Build history of the part. All positions in model axes, mm. Face numbers are marked on the shaded views. A direction names the side the tool comes from. Round coordinates to 2 decimals unless told otherwise and drop trailing zeros. Order: outer loops, then holes, each group sorted by start corner. A loop starts at its lowest first (then second) coordinate and runs counter-clockwise, first axis right, second up. Notation, with made-up numbers: (46, -38) -> (62, -38) arc R19 cw to (62, -10) -> close; hole circle Ø2 at (77.5, 21). An arc over 180 degrees is marked (long way). Answer as CSV lines item,"result". Start each with the question number.
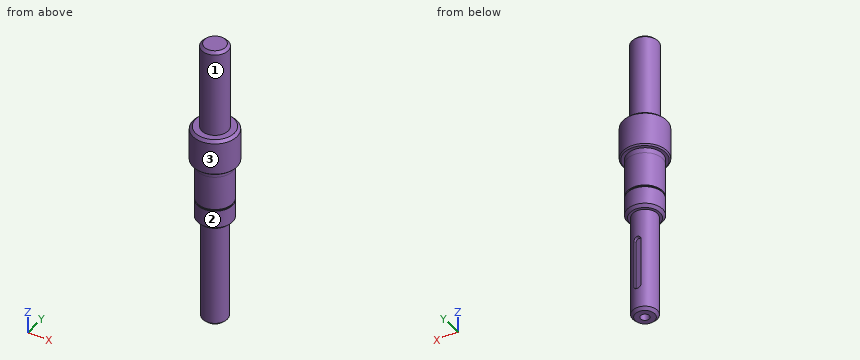
```python
from build123d import *

# Parameters (mm, degrees)
CHAMFER_1_SIZE         = 3
HOLE_WIZARD_M121_D     = 10.2
HOLE_WIZARD_M121_DEPTH = 30
HOLE_WIZARD_M121_TIP   = 3.064389157
SKETCH_4_R             = 20
SKETCH_4_R_2           = 18.75
CUT_EXTRUDE_1_DEPTH    = 2
FILLET_1_R             = 0.3
CHAMFER_2_SIZE         = 1.5
CUT_EXTRUDE_2_DEPTH    = 334.782863551
SKETCH_9_R             = 25
SKETCH_9_R_2           = 20
CUT_EXTRUDE_4_DEPTH    = 6
CHAMFER_3_SIZE         = 1.5
CHAMFER_4_SIZE         = 3


with BuildPart() as part:
    # Sketch 1 → Revolve 1 (revolve)
    with BuildSketch(Plane(origin=(0, 0, 0), x_dir=(0, 0, -1), z_dir=(1, 0, 0)), mode=Mode.PRIVATE) as revolve_1_sk:
        Polygon((0, 0), (0, 15), (100, 15), (100, 25), (147, 25), (147, 20), (211, 20), (211, 14), (331, 14), (331, 0), align=None)
    revolve(revolve_1_sk.sketch.rotate(Axis((0, 0, 0), (0, 0, -1)), 90), axis=Axis((0, 0, 0), (0, 0, -1)))

    # Chamfer 1
    chamfer_1_edges = [part.edges().sort_by_distance(p)[0] for p in [
        (-25, 0, -100),
        (-15, 0, 0),
        (-14, 0, -331),
    ]]
    chamfer(chamfer_1_edges, length=CHAMFER_1_SIZE)

    # Hole Wizard M121
    with Locations(Plane(origin=(0, 0, -331), x_dir=(-1, 0, 0), z_dir=(0, 0, -1))):
        with Locations((0, 0)):
            Hole(HOLE_WIZARD_M121_D / 2, depth=HOLE_WIZARD_M121_DEPTH)
            with Locations((0, 0, -(HOLE_WIZARD_M121_DEPTH + HOLE_WIZARD_M121_TIP / 2))):  # 118° drill point
                Cone(0, HOLE_WIZARD_M121_D / 2, HOLE_WIZARD_M121_TIP, mode=Mode.SUBTRACT)

    # Sketch 4 → Cut-Extrude 1 (cut)
    with BuildSketch(Plane(origin=(0, 0, -188), x_dir=(-1, 0, 0), z_dir=(0, 0, -1))):
        with Locations(Location((0, 0, 0), (0, 0, 180))):
            Circle(SKETCH_4_R)
        Circle(SKETCH_4_R_2, mode=Mode.SUBTRACT)
    extrude(amount=-CUT_EXTRUDE_1_DEPTH, mode=Mode.SUBTRACT)

    # Fillet 1
    fillet_1_edges = [part.edges().sort_by_distance(p)[0] for p in [
        (18.75, 0, -186),
        (18.75, 0, -188),
    ]]
    fillet(fillet_1_edges, radius=FILLET_1_R)

    # Chamfer 2
    chamfer_2_edges = [part.edges().sort_by_distance(p)[0] for p in [
        (-25, 0, -147),
    ]]
    chamfer(chamfer_2_edges, length=CHAMFER_2_SIZE)

    # Sketch 8 → Cut-Extrude 2 (cut, through all)
    with BuildSketch(Plane(origin=(0, 10, -331), x_dir=(-1, 0, 0), z_dir=(0, -1, 0))):
        with BuildLine():
            Line((4, -30), (4, -85))
            ThreePointArc((4, -85), (0, -89), (-4, -85))
            Line((-4, -85), (-4, -30))
            ThreePointArc((-4, -30), (0, -26), (4, -30))
        make_face()
    extrude(amount=-CUT_EXTRUDE_2_DEPTH, mode=Mode.SUBTRACT)

    # Sketch 9 → Cut-Extrude 4 (cut)
    with BuildSketch(Plane(origin=(0, 0, -147), x_dir=(-1, 0, 0), z_dir=(0, 0, -1))):
        Circle(SKETCH_9_R)
        Circle(SKETCH_9_R_2, mode=Mode.SUBTRACT)
    extrude(amount=-CUT_EXTRUDE_4_DEPTH, mode=Mode.SUBTRACT)

    # Chamfer 3
    chamfer_3_edges = [part.edges().sort_by_distance(p)[0] for p in [
        (-25, 0, -141),
    ]]
    chamfer(chamfer_3_edges, length=CHAMFER_3_SIZE)

    # Chamfer 4
    chamfer_4_edges = [part.edges().sort_by_distance(p)[0] for p in [
        (-20, 0, -211),
    ]]
    chamfer(chamfer_4_edges, length=CHAMFER_4_SIZE)


solid = part.part
```
Q1. Slice it at A-A, the plane z = -163.5. Write the cut outline in (x, y).
Q2. Flat gauge pins, fed straight in: pin 1 Ø2.5 at (y, z) = (12, -283.5) entering from -X; pin 2 Ø12 at (x, y) = (3, 15) entering from +Z; pin 3 Ø12 at (x, z) = (-19, -202) entering from -Y; pin 4 Ø8 at (y, z) = (14, -47) entering from +X. Where does each tip first touch, or does it go through?
Q3. Slice it at C-C, the plane z = -287. Write the cut outline in (x, y), plus the area to 3 significant figures.
Q4. Which spindle directions (+Z, -Z, +X, -X, +Y, -Y) get a long thin tool onto all of the face, cutting with end or side? Do the marked faces 1, 2 and 3. Say none if no direction does.
Q5. Probe L1, parallel to Y at x = 0, z = -321; L2, parallel to X at y = 1, z = -303.5; L3, parallel to Z at x = -12.5, y = -18. List the from-to ranges inside material, lowest first.
Q6. Slice it at B-B, the plane z = -71.5. Write the cut outline in (x, y), plus the area to 3 significant figures.
Solutions:
1,outline,"circle Ø40 at (0, 0)"
2,pin 1,"stops at x = -8.97"
2,pin 2,"stops at z = 0"
2,pin 3,"stops at y = -15.2"
2,pin 4,"stops at x = 11.18"
3,outline,"(-4, 10) -> (-4, 13.42) arc R14 ccw (long way) to (4, 13.42) -> (4, 10) -> close"
3,area,"585 mm2"
4,face 1,"+Z"
4,face 2,"-Z"
4,face 3,"+Z, -Z"
5,L1,"y = -14 to -5.1, 5.1 to 14"
5,L2,"x = -13.96 to -5, 5 to 13.96"
5,L3,"z = -141 to -100"
6,outline,"circle Ø30 at (0, 0)"
6,area,"707 mm2"
